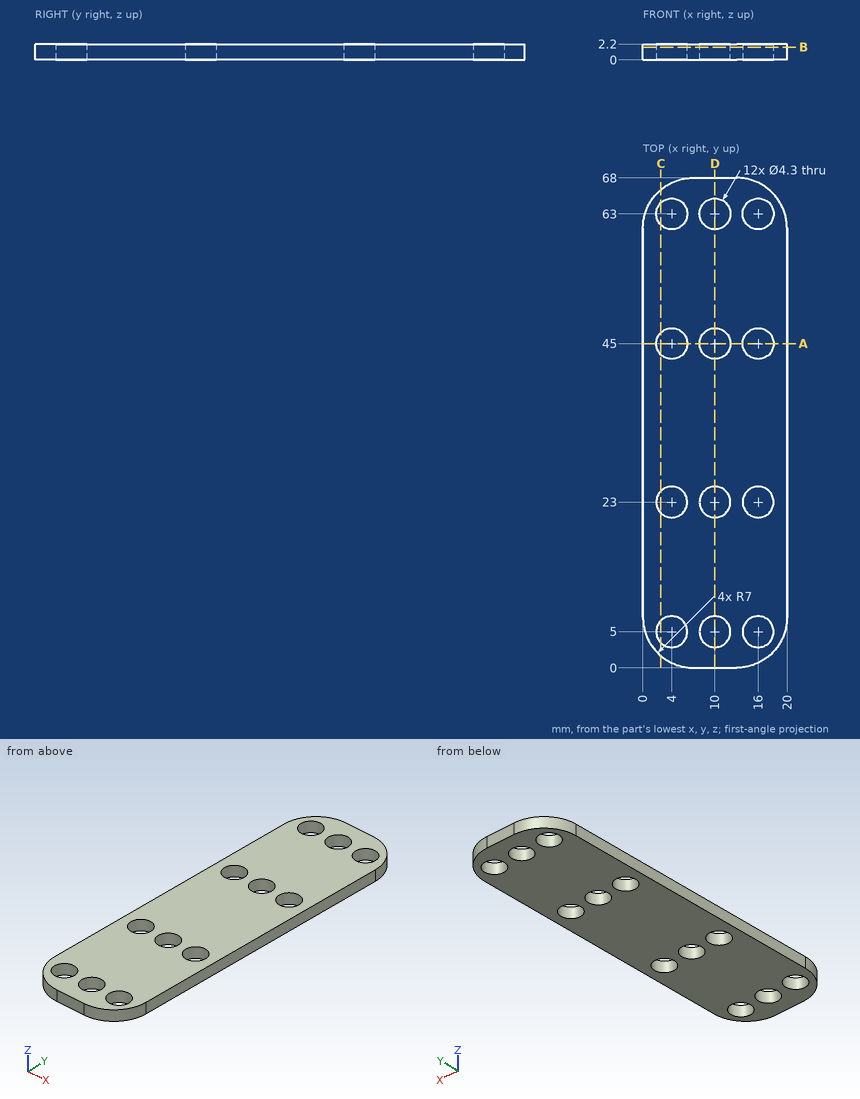
Study the drawing (mm; zero at the part's minimum x, y, z) and answer. Coordinates: 2 decimals unless noted, no trailing zeros. Loops run counter-clockwise (first coordinate to the right, second up) from the corner with the lowest first, then second, coordinate; pieces in that order, holes last. Notation, with made-up numbers: M 36.5,53.5 L 94.5,53.5 A33 cw 94.5,86.5 Z; hole C 66,3 d3. An arc over 180 degrees is marked long. Answer in a Markdown table with one row per item. Add a question column.
1. Find section A-A, the plane y = 45. Write down the section's boundary in (x, z), then the cut area to 3 significant figures.
2. Consider L1, parallel to X at y = 45, z = 1.2; L2, parallel to Y at x = 10, z = 0.4; L3, parallel to Y at x = 4, z = 1.1. Determine where each line is inside the solid, lowest interval first.
3. Find section B-B, the plane z = 1.75. State how many separate pieces and enclosed holes the cut face has, then the cut area to 3 significant figures.
4. Find section C-C, the plane x = 2.5. Write down the section's boundary in (y, z), then the cut area to 3 significant figures.
5. A flat-ended cylindrical pin translates along its axis: P1, Ø4, axis at x = 4, y = 23, coming from the +Z side. Find the tip coordinate at first contact, or state that the pin passes through.
6. Find section D-D, the plane x = 10. Write down the section's boundary in (y, z), then the cut area to 3 significant figures.
Reported:
| question | item | result |
|---|---|---|
| 1 | outline | M 0,0 L 1.85,0 L 1.85,2.2 L 0,2.2 Z; M 6.15,0 L 7.85,0 L 7.85,2.2 L 6.15,2.2 Z; M 12.15,0 L 13.85,0 L 13.85,2.2 L 12.15,2.2 Z; M 18.15,0 L 20,0 L 20,2.2 L 18.15,2.2 Z |
| 1 | area | 15.6 mm^2 |
| 2 | L1 | x = 0 to 1.85, 6.15 to 7.85, 12.15 to 13.85, 18.15 to 20 |
| 2 | L2 | y = 0 to 2.85, 7.15 to 20.85, 25.15 to 42.85, 47.15 to 60.85, 65.15 to 68 |
| 2 | L3 | y = 0.68 to 2.85, 7.15 to 20.85, 25.15 to 42.85, 47.15 to 60.85, 65.15 to 67.32 |
| 3 | separate pieces | 1 |
| 3 | enclosed holes | 12 |
| 3 | area | 1,140 mm^2 |
| 4 | outline | M 1.64,0 L 3.46,0 L 3.46,2.2 L 1.64,2.2 Z; M 6.54,0 L 21.46,0 L 21.46,2.2 L 6.54,2.2 Z; M 24.54,0 L 43.46,0 L 43.46,2.2 L 24.54,2.2 Z; M 46.54,0 L 61.46,0 L 61.46,2.2 L 46.54,2.2 Z; M 64.54,0 L 66.36,0 L 66.36,2.2 L 64.54,2.2 Z |
| 4 | area | 115 mm^2 |
| 5 | P1 | passes through |
| 6 | outline | M 0,0 L 2.85,0 L 2.85,2.2 L 0,2.2 Z; M 7.15,0 L 20.85,0 L 20.85,2.2 L 7.15,2.2 Z; M 25.15,0 L 42.85,0 L 42.85,2.2 L 25.15,2.2 Z; M 47.15,0 L 60.85,0 L 60.85,2.2 L 47.15,2.2 Z; M 65.15,0 L 68,0 L 68,2.2 L 65.15,2.2 Z |
| 6 | area | 112 mm^2 |
